from build123d import *

# Parameters (mm, degrees)
SKETCH1_R           = 2.025
BOSS_EXTRUDE1_DEPTH = 2
FILLET1_R           = 3


with BuildPart() as part:
    # Sketch1 → Boss-Extrude1 (new body)
    with BuildSketch(Plane.XY):
        Polygon((-24, 15), (-16.452815094, 15), (0, 4.716990566), (16.452815094, 15), (24, 15), (24, 10.283009434), (7.547184906, 0), (24, -10.283009434), (24, -15), (16.452815094, -15), (0, -4.716990566), (-16.452815094, -15), (-24, -15), (-24, -10.283009434), (-7.547184906, 0), (-24, 10.283009434), align=None)
        with Locations((-16, 10)):
            Circle(SKETCH1_R, mode=Mode.SUBTRACT)
        with Locations((16, 10)):
            Circle(SKETCH1_R, mode=Mode.SUBTRACT)
        with Locations((16, -10)):
            Circle(SKETCH1_R, mode=Mode.SUBTRACT)
        with Locations((-16, -10)):
            Circle(SKETCH1_R, mode=Mode.SUBTRACT)
    extrude(amount=BOSS_EXTRUDE1_DEPTH)

    # Fillet1
    fillet1_edges = [part.edges().sort_by_distance(p)[0] for p in [
        (24, -15, 1),
        (0, -4.716990566, 1),
        (-24, -15, 1),
        (-7.547184906, 0, 1),
        (-24, 15, 1),
        (0, 4.716990566, 1),
        (24, 15, 1),
        (7.547184906, 0, 1),
    ]]
    fillet(fillet1_edges, radius=FILLET1_R)


solid = part.part
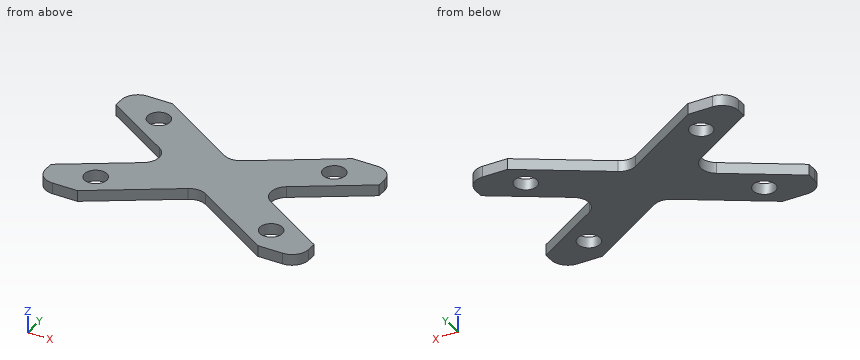
Model file for the job. Use its own axes, mm. Round coordinates to 2 decimals unless told otherwise and drop trailing zeros. Loops run counter-clockwise (first coordinate to the right, second up) from the corner with the lowest first, then second, coordinate; pieces in that order, holes last. Notation, with made-up numbers: (-19, 39) -> (4, 39) arc R12 cw to (4, 48) -> close; hole circle Ø1 at (74.25, 84.5). An arc over 180 degrees is marked (long way). Answer as CSV lines item,"result". Start each with the question number.
1) Slice it at A-A (z = 0.55). List the corners of the cut face in (x, y) (3 decimals), plus the area to 3 significant figures.
2) Probe line 1 along Y through (x, z) = (-16, 0.65) (3 decimals); line 2 along X through (y, z) = (8.25, 1.45); line 3 along Y through (x, z) = (11, 1.55). List the from-to ranges inside material, lowest first.
3) Slice it at D-D (y = 1.25). List the corners of the cut face in (x, z).
4) Pin check, flat tip, straight feed: P1, Ø1, axis at x = -14.5, z = 1.5, coming from the +Y side. Stop position of the tip, or through.
5) Slice it at C-C (y = -3). List the corners of the cut face in (x, z), plus the area to 3 significant figures.
6) Slice it at B-B (y = 10.75). List the corners of the cut face in (x, z), plus the area to 3 significant figures.
Filled in:
1,outline,"(-24, -12) arc R3 ccw to (-21, -15) -> (-16.453, -15) -> (-1.59, -5.711) arc R3 cw to (1.59, -5.711) -> (16.453, -15) -> (21, -15) arc R3 ccw to (24, -12) -> (24, -10.283) -> (11.618, -2.544) arc R3 cw to (11.618, 2.544) -> (24, 10.283) -> (24, 12) arc R3 ccw to (21, 15) -> (16.453, 15) -> (1.59, 5.711) arc R3 cw to (-1.59, 5.711) -> (-16.453, 15) -> (-21, 15) arc R3 ccw to (-24, 12) -> (-24, 10.283) -> (-11.618, 2.544) arc R3 cw to (-11.618, -2.544) -> (-24, -10.283) -> close; hole circle Ø4.05 at (-16, -10); hole circle Ø4.05 at (-16, 10); hole circle Ø4.05 at (16, -10); hole circle Ø4.05 at (16, 10)"
1,area,"716 mm2"
2,line 1,"y = -14.717 to -12.025, -7.975 to -5.283, 5.283 to 7.975, 12.025 to 14.717"
2,line 2,"x = -20.75 to -17.02, -14.98 to -5.65, 5.65 to 14.98, 17.02 to 20.75"
2,line 3,"y = -11.59 to -2.03, 2.03 to 11.59"
3,outline,"(-10.48, 0) -> (10.48, 0) -> (10.48, 2) -> (-10.48, 2) -> close"
4,P1,"stops at y = 14.09"
5,outline,"(-12.35, 0) -> (12.35, 0) -> (12.35, 2) -> (-12.35, 2) -> close"
5,area,"49.4 mm2"
6,outline,"(-24, 0) -> (-17.88, 0) -> (-17.88, 2) -> (-24, 2) -> close; (-14.12, 0) -> (-9.65, 0) -> (-9.65, 2) -> (-14.12, 2) -> close; (9.65, 0) -> (14.12, 0) -> (14.12, 2) -> (9.65, 2) -> close; (17.88, 0) -> (24, 0) -> (24, 2) -> (17.88, 2) -> close"
6,area,"42.3 mm2"
